Check sheet for the modelled part. Datum: model origin and axes. Units: mm. Face numbers are marked on the shaded views. A direction names the side the tool comes from. Coordinates: 2 decimals unless noted, no trailing zeros. Loops run counter-clockwise (first coordinate to the right, second up) from the corner with the lowest first, then second, coordinate; pieces in that order, holes last. Notation, with made-up numbers: M 29.5,-30.5 L 49.5,-30.5 A10 ccw 49.5,-19.5 Z; hole C 47,-31 d4. An arc over 180 degrees is marked long. Return JSON: item names as keys, results as strings.
Autodesk Inventor part; units mm, degrees
ref_plane "YZ Plane" through (0, 0, 0) normal (1, 0, 0) x (0, 1, 0)
ref_plane "XZ Plane" through (0, 0, 0) normal (0, 1, 0) x (-1, 0, 0)
ref_plane "XY Plane" through (0, 0, 0) normal (0, 0, 1) x (1, 0, 0)
sketch "スケッチ1" plane through (0, 0, 0) normal (0, 1, 0) x (-1, 0, 0)
  circle A0 centre (0, 0) radius 20
  circle A1 centre (0, 0) radius 29
  arc A2 (31.7208, -14.7916) -> (31.7208, 14.7916) centre (0, 0) ccw
  line L0 (0, 0) -> (31.7208, 14.7916) construction
  line L1 (0, 0) -> (35, 0) construction
  line L2 (0, 0) -> (31.7208, -14.7916) construction
  arc A3 (-31.7129, 14.8084) -> (-31.7208, -14.7915) centre (0, 0) ccw
  circle A4 centre (0.0475, 45) radius 6.5
  circle A5 centre (-0.0487, -45) radius 6.5
  arc A6 (13.9039, 53) -> (-13.8089, 53) centre (0.0475, 45) ccw
  line L3 (0.0475, 45) -> (13.9039, 53) construction
  line L4 (0.0475, 45) -> (16.0475, 45) construction
  line L5 (0.0475, 45) -> (-13.8089, 53) construction
  arc A7 (-13.8991, -53.0102) -> (13.8137, -52.9897) centre (-0.0487, -45) ccw
  line L6 (-0.0487, -45) -> (-13.8991, -53.0102) construction
  line L7 (-0.0487, -45) -> (13.8137, -52.9897) construction
  line L8 (13.9039, 53) -> (31.7208, 14.7916)
  line L9 (-13.8089, 53) -> (-31.7129, 14.8084)
  line L10 (-31.7208, -14.7915) -> (-13.8991, -53.0102)
  line L11 (13.8137, -52.9897) -> (31.7208, -14.7916)
  dimension "d0" = 40
  dimension "d1" = 58
  dimension "d2" = 35
  dimension "d3" = 25
  dimension "d4" = 50
  dimension "d5" = 35
  dimension "d6" = 13
  dimension "d7" = 13
  dimension "d8" = 45
  dimension "d9" = 45
  dimension "d10" = 16
  dimension "d11" = 30
  dimension "d12" = 120
  dimension "d13" = 16
  dimension "d14" = 120
extrude "押し出し1" add sketch "スケッチ1" along normal blind 10 contours A1 | L11 A7 L10 A3 L9 A6 L8 A2
sketch "スケッチ2" plane through (0, 0, 0) normal (0, -1, 0) x (1, 0, 0)
  circle A0 centre (0, 0) radius 29
  circle A1 centre (0, 0) radius 20
  dimension "d17" = 58
extrude "押し出し2" add sketch "スケッチ2" along normal blind 20
chamfer "面取り1" distance 9 angle 15 1 edges at (-20, -20, 0) measured on face at (25.5254, -20, -3.9088)
fillet "フィレット1" radius 2 1 edges at (-29, 0, 0)
properties part number "パッキン押え"
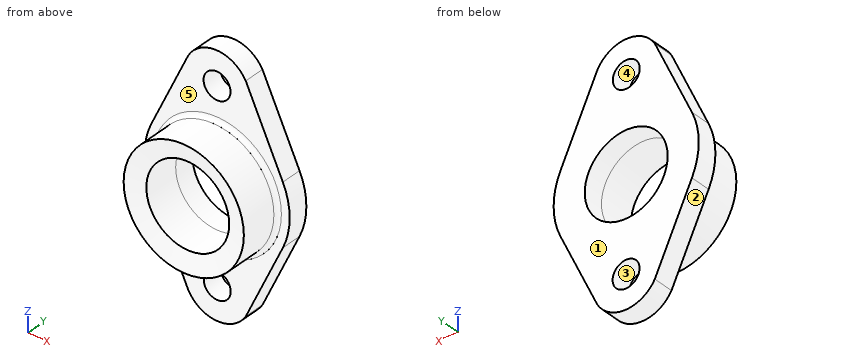
1) Go/stop test with flat-tipped pins: pin 1 Ø2 at (x, y) = (9, -15) entering from +Z; pin 2 Ø10 at (y, z) = (6.5, -16.5) entering from -X; pin 3 Ø1.5 at (y, z) = (-13, 20) entering from +X. Record where each tip stops, or that it passes through.
Answers:
{"pin 1": "z = 27.87", "pin 2": "x = -33.06", "pin 3": "x = 21.69"}
2) Section check B-B on x = 0. Count the separate pieces of the cut face and the enclosed holes in it, then the cut area to 3 significant figures.
Answers:
{"separate pieces": "4", "enclosed holes": "0", "area": "900 mm²"}
3) Section check D-D on y = -11.25. Record the cut outline in (x, z).
Answers:
{"outline": "C 0,0 d58; hole C 0,0 d40"}
4) Draft check along X on the marked faces 1, 2 and 3. Enter one of: +X half, -X half, draft (parallel to the pull), parting line (faces both ways), or undercut.
Answers:
{"face 1": "draft", "face 2": "-X half", "face 3": "undercut"}
5) Scan lines: line 1 along X through (y, z) = (-7.75, 0.5); line 2 along Y through (x, z) = (11, 49); line 3 along Z through (x, y) = (-13.5, -3). Record each from-to range of solid material in increasing order. Write a range as [from, to].
Answers:
{"line 1": "[-29, -19.99], [19.99, 29]", "line 2": "[0, 10]", "line 3": "[-25.67, -14.76], [14.76, 25.67]"}
6) Set-up check for the marked faces 4 and 5: record each of +Z, -Z, +X, -X, +Y, -Y from which the full face is reachable in a straight line by a thin tool's end or side.
Answers:
{"face 4": "+Y, -Y", "face 5": "-Y"}
7) Section check A-A on y = 4.75. Record the cut outline in (x, z).
Answers:
{"outline": "M -31.72,-14.79 L -13.81,-52.99 A16 ccw 13.9,-53.01 L 31.72,-14.79 A35 ccw 31.71,14.81 L 13.81,53 A16 ccw -13.9,53 L -31.72,14.79 A35 ccw Z; hole C 0,0 d40; hole C -0.05,45 d13; hole C 0.05,-45 d13"}
